Part model, mm, in its own coordinate system. A direction names the side the tool comes from. Coordinates: 2 decimals unless noted, no trailing zeros.
from build123d import *


with BuildPart() as f3:
    # F0 (on Right) → F3 section 0
    with BuildSketch(Plane.YZ):
        with BuildLine():
            Line((-135, 0), (-115, 0))
            ThreePointArc((-115, 0), (0, -40), (115, 0))
            Line((115, 0), (135, 0))
            Line((135, 0), (135, 0.8))
            Line((135, 0.8), (114.7214016651, 0.8))
            ThreePointArc((114.7214016651, 0.8), (0, -39.2), (-114.7214016651, 0.8))
            Line((-114.7214016651, 0.8), (-135, 0.8))
            Line((-135, 0.8), (-135, 0))
        make_face()
    # F2 (on offset) → F3 section 1
    with BuildSketch(Plane.YZ.offset(200)):
        with BuildLine():
            Line((-135, 0), (-115, 0))
            ThreePointArc((-115, 0), (0, -80), (115, 0))
            Line((115, 0), (135, 0))
            Line((135, 0), (135, 0.8))
            Line((135, 0.8), (114.4421251113, 0.8))
            ThreePointArc((114.4421251113, 0.8), (0, -79.2), (-114.4421251113, 0.8))
            Line((-114.4421251113, 0.8), (-135, 0.8))
            Line((-135, 0.8), (-135, 0))
        make_face()
    loft()


solid = f3.part
Q1. Which spindle directions (+Z, -Z, +X, -X, +Y, -Y) get a long thin tool onto all of the face, cutting with end or side? Do faces 1 (the face through (101, 125, 0)), 2 (the face through (101, -125, 0)). Say none if no direction does.
Results list:
face 1: -Z, +X, -X, +Y
face 2: -Z, +X, -X, -Y
Q2. Pin check, flat tips, straight feed: pin 1 Ø1.5 at (x, y) = (121.5, -17.5) entering from +Z; pin 2 Ø2 at (x, y) = (21, 87) entering from +Z; pin 3 Ø5 at (x, z) = (71.5, -44) entering from -Y. Stop position of each tip, or through.
Results list:
pin 1: stops at z = -62.18
pin 2: stops at z = -19.01
pin 3: stops at y = -60.62
Q3. Wall check: line 1 along Y through (x, z) = (83.5, -14.5); line 2 along Y through (x, z) = (116.5, -50); line 3 along Z through (x, y) = (162.5, -112) (3 decimals). Give the ranges that are in metal, low to high.
Results list:
line 1: y = -102.35 to -101.22, 101.22 to 102.35
line 2: y = -58.86 to -56.98, 56.98 to 58.86
line 3: z = -5.945 to -4.244
